Can you work these out from the model? Positions are in its coordinate system, mm. A direction names the side the tool comes from. Coordinates: 2 decimals unless noted, no trailing zeros. Write each loop counter-clockwise with the first axis right and the second up, starting at its lowest first coordinate (ties: lowest second). Pieces come first, ordered by that corner, then holes. Notation, with made-up numbers: (23.25, 10) - (68.25, 10) arc R16 cw to (68.25, 17) - close; hole circle Ø10 at (72, 82). An arc over 180 degrees is marked (long way). Use one line per item in the form item = value. Start each with the question number.
(1) For pin 1 Ø0.9 at (y, z) = (35.5, 1) entering from -X; pin 2 Ø1.5 at (y, z) = (27, 1) entering from +X, each with a flat end and sliding along its axis, tell me the tip position at first contact or that it passes through.
(2) If we section it at B-B on z = 1: Give the number of separate pieces and of enclosed holes in the cut face, then the cut area to 3 significant figures.
(3) If we section it at C-C on y = 42: Please give me the cut outline in (x, z).
(4) On a 3-axis mill with a long thin cutter (end or side, diameter ignored), from which of +Z, -Z, +X, -X, +Y, -Y can I reach the whole of each face in a straight line? I mean faces 1 (the face through (0, 48.6, 2)), 2 (the face through (0, 24, 3)). Say none if no direction works.
(5) If I drill on probe 1 along X at (y, z) = (26.5, 2.3); probe 2 along X at (y, z) = (41, 0.3); probe 3 along X at (y, z) = (35.5, 1.75), over which ranges is the centre line in solid material (lowest first)? Write a range as from..to.
(6) If we section it at A-A on y = 28: Please give me the cut outline in (x, z), then the cut area to 3 significant figures.
(7) Thinking about a two-plate mould opening in X: for faces 3 (the face through (0, 24, 0)), 4 (the face through (-0.13, -7.49, 1.48)), 5 (the face through (0, 24.6, 2)), 6 (the face through (7, 31, 1)), which applies, pulls with the +X half, pulls with the -X half, needs draft (parallel to the pull), parting line crosses it, or undercut?
```python
from build123d import *

# Parameters (mm, degrees)
SKETCH_1_W               = 14
SKETCH_1_H               = 13.200286042
EXTRUDE_1_DEPTH          = 3
SKETCH_3_OUTSIDE_W       = 35.048
SKETCH_3_OUTSIDE_H       = 82.027
CUT_EXTRUDE_2_DEPTH      = 3
SKETCH_4_R               = 3
CUT_EXTRUDE_3_DEPTH      = 10
SKETCH_5_R               = 1
CUT_EXTRUDE_4_DEPTH      = 10
SKETCH_6_W               = 4
SKETCH_6_H               = 4
EXTRUDE_3_DEPTH          = 3
CUT_EXTRUDE_5_DEPTH      = 10
PATTERN_CIRCULAR_1_COUNT = 8


with BuildPart() as part:
    # 草图1 → 凸台-拉伸1 (new body)
    with BuildSketch(Plane.XY):
        Rectangle(SKETCH_1_W, SKETCH_1_H)
        with BuildLine():
            ThreePointArc((-7, 6.600143021), (-9.620908892, 0), (-7, -6.600143021))
            Line((-7, -6.600143021), (-7, 6.600143021))
        make_face()
        with BuildLine():
            Line((7, -6.600143021), (-7, -6.600143021))
            ThreePointArc((-7, -6.600143021), (0, -9.620908892), (7, -6.600143021))
        make_face()
        with BuildLine():
            Line((7, 6.600143021), (7, -6.600143021))
            ThreePointArc((7, -6.600143021), (8.941707056, -3.550741166), (9.620908892, 0))
            ThreePointArc((9.620908892, 0), (8.941707056, 3.550741166), (7, 6.600143021))
        make_face()
        with BuildLine():
            ThreePointArc((7, 6.600143021), (0, 9.620908892), (-7, 6.600143021))
            Line((-7, 6.600143021), (7, 6.600143021))
        make_face()
        with BuildLine():
            Line((-7, 56.600143021), (-7, 6.600143021))
            ThreePointArc((-7, 6.600143021), (0, 9.620908892), (7, 6.600143021))
            Line((7, 6.600143021), (7, 56.600143021))
            Line((7, 56.600143021), (-7, 56.600143021))
        make_face()
    extrude(amount=EXTRUDE_1_DEPTH)

    # 草图3 outside → 切除-拉伸2 (cut)
    with BuildSketch(Plane.XY.offset(3)):
        with Locations((0, 23.4895)):
            Rectangle(SKETCH_3_OUTSIDE_W, SKETCH_3_OUTSIDE_H)
        with BuildLine():
            Line((7, 56.600143021), (0, 56.600143021))
            Line((0, 56.600143021), (-7, 56.600143021))
            Line((-7, 56.600143021), (-7, 6.600143021))
            ThreePointArc((-7, 6.600143021), (0, -9.620908892), (7, 6.600143021))
            Line((7, 6.600143021), (7, 56.600143021))
        make_face(mode=Mode.SUBTRACT)
        Polygon((-2, 28.600143021), (0, 28.600143021), (2, 28.600143021), (2, 24.600143021), (-2, 24.600143021), align=None)
        Polygon((-2, 38.600143021), (0, 38.600143021), (2, 38.600143021), (2, 34.600143021), (0, 34.600143021), (-2, 34.600143021), align=None)
        Polygon((-2, 48.600143021), (0, 48.600143021), (2, 48.600143021), (2, 44.600143021), (0, 44.600143021), (-2, 44.600143021), align=None)
    extrude(amount=-CUT_EXTRUDE_2_DEPTH, mode=Mode.SUBTRACT)

    # 草图4 → 切除-拉伸3 (cut)
    with BuildSketch(Plane.XY.offset(3)):
        Circle(SKETCH_4_R)
    extrude(amount=-CUT_EXTRUDE_3_DEPTH, mode=Mode.SUBTRACT)

    # 草图5 → 切除-拉伸4 (cut)
    with BuildSketch(Plane(origin=(0, 0, 0), x_dir=(-1, 0, 0), z_dir=(0, 0, -1))):
        with Locations((0, 6.5)):
            Circle(SKETCH_5_R)
    cut_extrude_4 = extrude(amount=-CUT_EXTRUDE_4_DEPTH, mode=Mode.SUBTRACT)

    # 草图6 → 凸台-拉伸3 (add)
    with BuildSketch(Plane(origin=(0, 0, 0), x_dir=(-1, 0, 0), z_dir=(0, 0, -1))):
        with Locations((0, 36.600143021)):
            Rectangle(SKETCH_6_W, SKETCH_6_H)
    extrude(amount=-EXTRUDE_3_DEPTH)

    # 草图7 → 切除-拉伸5 (cut)
    with BuildSketch(Plane(origin=(0, 0, 0), x_dir=(-1, 0, 0), z_dir=(0, 0, -1))):
        with BuildLine():
            ThreePointArc((0, 38.600143021), (-2, 36.600143021), (0, 34.600143021))
            Line((0, 34.600143021), (0, 38.600143021))
        make_face()
        with BuildLine():
            Line((0, 38.600143021), (0, 34.600143021))
            ThreePointArc((0, 34.600143021), (1.414213562, 35.185929459), (2, 36.600143021))
            ThreePointArc((2, 36.600143021), (1.414213562, 38.014356584), (0, 38.600143021))
        make_face()
    extrude(amount=-CUT_EXTRUDE_5_DEPTH, mode=Mode.SUBTRACT)

    # 阵列(圆周)1: 切除-拉伸4 ×8 about axis
    pattern_circular_1_axis = Axis((0, 0, 0), (0, 0, 1))
    for i in range(1, PATTERN_CIRCULAR_1_COUNT):
        add(cut_extrude_4.rotate(pattern_circular_1_axis, i * 360 / PATTERN_CIRCULAR_1_COUNT), mode=Mode.SUBTRACT)


solid = part.part
```
Reported:
q1.pin_1 = -7
q1.pin_2 = 7
q2.separate_pieces = 1
q2.enclosed_holes = 12
q2.area = 864 mm2
q3.outline = (-7, 0) - (7, 0) - (7, 3) - (-7, 3) - close
q4.face_1 = +Z, -Z
q4.face_2 = +Z, +X, -X, +Y, -Y
q5.probe_1 = -7..-2, 2..7
q5.probe_2 = -7..7
q5.probe_3 = -7..-1.67, 1.67..7
q6.outline = (-7, 0) - (-2, 0) - (-2, 3) - (-7, 3) - close; (2, 0) - (7, 0) - (7, 3) - (2, 3) - close
q6.area = 30.0 mm2
q7.face_3 = needs draft
q7.face_4 = undercut
q7.face_5 = undercut
q7.face_6 = pulls with the +X half
